Here's how the part is built. I have some questions about the finished solid (model axes, mm). Round coordinates to 2 decimals unless told otherwise and drop trailing zeros. Order: outer loops, then holes, each group sorted by start corner. A loop starts at its lowest first (then second) coordinate and runs counter-clockwise, first axis right, second up.
```python
from build123d import *

# Parameters (mm, degrees)
SKETCH_1_W          = 250
SKETCH_1_H          = 60
EXTRUDE_2_DEPTH     = 44.32
FILLET_2_RADIUS     = 30
FILLET_2_LENGTH     = 44.32
SKETCH_2_R          = 1
EXTRUDE_3_DEPTH     = 3
SKETCH_3_R          = 2
CUT_EXTRUDE_1_DEPTH = 44.32
SKETCH_4_R          = 4
CUT_EXTRUDE_2_DEPTH = 103


with BuildPart() as part:
    # 草图1 → 凸台-拉伸2 (new body)
    with BuildSketch(Plane(origin=(0, 0, 0), x_dir=(0, 0, -1), z_dir=(1, 0, 0))):
        Rectangle(SKETCH_1_W, SKETCH_1_H)
    extrude(amount=EXTRUDE_2_DEPTH)

    # 圆角2: full round fillet: the end face becomes a half cylinder, R = half its width
    fillet_2_face = Plane((22.16, 0, 125), x_dir=(1, 0, 0), z_dir=(0, 0, 1))  # on the end face: x along it, z out of the body
    fillet_2_slab = fillet_2_face.offset(-FILLET_2_RADIUS / 2) * Box(FILLET_2_LENGTH, 2 * FILLET_2_RADIUS, FILLET_2_RADIUS, mode=Mode.PRIVATE)  # the body's end, R deep
    fillet_2_round = Plane((22.16, 0, 95), x_dir=(0, 0, 1), z_dir=(1, 0, 0)) * Cylinder(FILLET_2_RADIUS, FILLET_2_LENGTH, mode=Mode.PRIVATE)  # its axis R under the face
    add(fillet_2_slab - fillet_2_round, mode=Mode.SUBTRACT)

    # 草图2 → 凸台-拉伸3 (add)
    with BuildSketch(Plane(origin=(0, 0, -125), x_dir=(-1, 0, 0), z_dir=(0, 0, -1))):
        with Locations(Location((-22.436932243, 0, 0), (0, 0, 270))):
            Circle(SKETCH_2_R)
    extrude(amount=EXTRUDE_3_DEPTH)

    # 草图3 → 切除-拉伸1 (cut)
    with BuildSketch(Plane.ZY):
        with Locations((95, 17.25)):
            Circle(SKETCH_3_R)
        with Locations((109.938938215, 8.625)):
            Circle(SKETCH_3_R)
        with Locations((109.938938215, -8.625)):
            Circle(SKETCH_3_R)
        with Locations((95, -17.25)):
            Circle(SKETCH_3_R)
        with Locations((80.061061785, -8.625)):
            Circle(SKETCH_3_R)
        with Locations((80.061061785, 8.625)):
            Circle(SKETCH_3_R)
    extrude(amount=-CUT_EXTRUDE_1_DEPTH, mode=Mode.SUBTRACT)

    # 草图4 → 切除-拉伸2 (cut)
    with BuildSketch(Plane.ZY):
        with Locations((95, 0)):
            Circle(SKETCH_4_R)
    extrude(amount=-CUT_EXTRUDE_2_DEPTH, mode=Mode.SUBTRACT)


solid = part.part
```
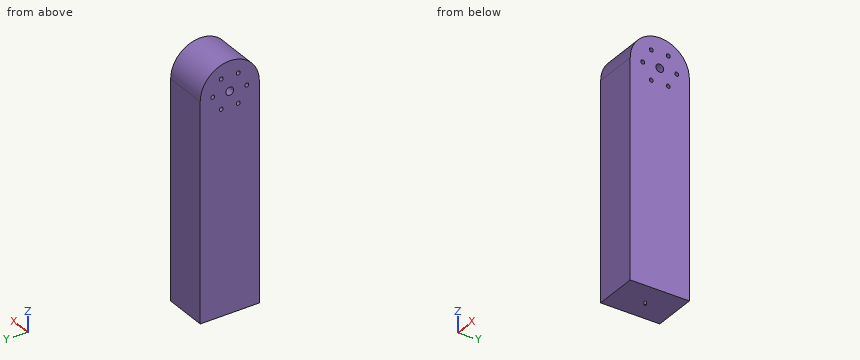
1) If we section it at B-B (y = 22.5): Write out the boundary of the cut face in (x, z).
2) I need wall thicknesses on line 1 (Y direction, x = 11, z = 95); line 2 (Y direction, x = 21.5, z = 110.5); line 3 (Z direction, x = 10, y = -8). Which ranges of each line are inside material? Lowest first, please.
3) If we section it at A-A (x = 31.5): Write out the boundary of the cut face in (y, z) (3 decimals), plus the area to 3 significant figures.
4) I'm going to push flat-ended pins straight in: pin 1 (6.5 mm diameter, centred on y = 8.62, z = 109.94, fed in from +X); pin 2 (4 mm diameter, centred on x = 16, y = 5.5, fed in from -Z). Where does each tip first touch, or does it pass through?
Solutions:
1. outline: (0, -125) - (44.32, -125) - (44.32, 114.84) - (0, 114.84) - close
2. line 1: y = -30 to -19.25, -15.25 to -4, 4 to 15.25, 19.25 to 30
2. line 2: y = -25.69 to -10.54, -6.71 to 6.71, 10.54 to 25.69
2. line 3: z = -125 to 78.16, 81.96 to 108.04, 111.84 to 123.91
3. outline: (-30, -125) - (30, -125) - (30, 95) arc R30 ccw to (-30, 95) - close; hole circle Ø4 at (-17.25, 95); hole circle Ø4 at (-8.625, 80.061); hole circle Ø4 at (-8.625, 109.939); hole circle Ø8 at (0, 95); hole circle Ø4 at (8.625, 80.061); hole circle Ø4 at (8.625, 109.939); hole circle Ø4 at (17.25, 95)
3. area: 14,500 mm2
4. pin 1: stops at x = 44.32
4. pin 2: stops at z = -125
